Check sheet for the modelled part. Datum: model origin and axes. Units: mm. Coordinates: 2 decimals unless noted, no trailing zeros. Loops run counter-clockwise (first coordinate to the right, second up) from the corner with the lowest first, then second, coordinate; pieces in that order, holes last. Notation, with made-up numbers: (63, 21.5) -> (119, 21.5) arc R33 ccw to (119, 55.5) -> close; hole circle Ø8 at (-12.75, 6.5). An arc over 180 degrees is marked (long way). Use one line per item in the form item = value.
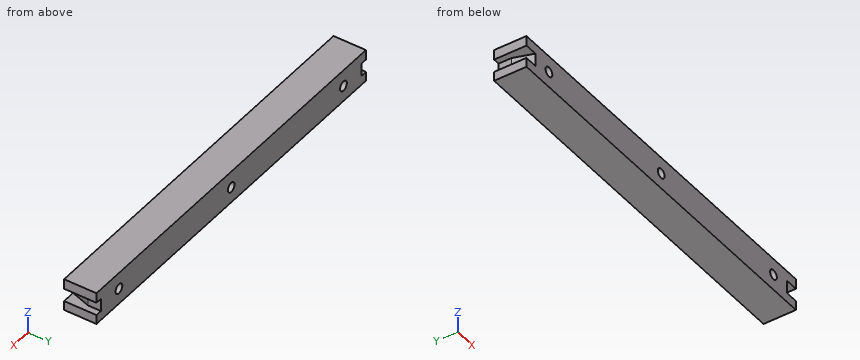
from build123d import *

# Parameters (mm, degrees)
ESQUISSE1_W                  = 120
ESQUISSE1_H                  = 10
ESQUISSE1_R                  = 1.5
BOSS_EXTRU_1_DEPTH           = 10
ENL_V_MAT_EXTRU_1_DEPTH      = 2
ENL_V_MAT_EXTRU_1_DEPTH_BACK = 2


with BuildPart() as part:
    # Esquisse1 → Boss.-Extru.1 (new body)
    with BuildSketch(Plane(origin=(0, 0, 0), x_dir=(1, 0, 0), z_dir=(0, 1, 0))):
        with Locations((0, -0.107913669)):
            Rectangle(ESQUISSE1_W, ESQUISSE1_H)
        with Locations((-50, 0)):
            Circle(ESQUISSE1_R, mode=Mode.SUBTRACT)
        Circle(ESQUISSE1_R, mode=Mode.SUBTRACT)
        with Locations((50, 0)):
            Circle(ESQUISSE1_R, mode=Mode.SUBTRACT)
    extrude(amount=BOSS_EXTRU_1_DEPTH)

    # Esquisse2 → Enlèv. mat.-Extru.1 (cut, two sides)
    with BuildSketch(Plane.XY) as enl_v_mat_extru_1_sk:
        Polygon((-58, 10), (-58, 6), (-56, 0), (-56, -10.800752999), (-73.153181154, -10.800752999), (-73.153181154, 18.339979991), (-58, 18.339979991), align=None)
        Polygon((58, 10), (58, 6), (56, 0), (56, -10.800752999), (73.153181154, -10.800752999), (73.153181154, 18.339979991), (58, 18.339979991), align=None)
    extrude(amount=ENL_V_MAT_EXTRU_1_DEPTH, mode=Mode.SUBTRACT)
    extrude(enl_v_mat_extru_1_sk.sketch, amount=-ENL_V_MAT_EXTRU_1_DEPTH_BACK, mode=Mode.SUBTRACT)


solid = part.part
(1) Section check B-B, the plane z = 0. Record the boundary of the cut face in (x, y), plus the area to 3 significant figures.
Established:
outline = (-58, 6) -> (-56, 0) -> (-51.5, 0) -> (-51.5, 10) -> (-58, 10) -> close; (-48.5, 0) -> (-1.5, 0) -> (-1.5, 10) -> (-48.5, 10) -> close; (1.5, 0) -> (48.5, 0) -> (48.5, 10) -> (1.5, 10) -> close; (51.5, 0) -> (56, 0) -> (58, 6) -> (58, 10) -> (51.5, 10) -> close
area = 1,060 mm²
(2) Go/stop test with a flat-tipped pin: P1, Ø2.5, axis at x = 0, z = 0, coming from the -Y side. Record where the tip stops, or that it passes through.
Established:
P1 = through
(3) Section check C-C, the plane y = 7. Record the boundary of the cut face in (x, z), plus the area to 3 significant figures.
Established:
outline = (-60, -4.89) -> (60, -4.89) -> (60, -2) -> (58, -2) -> (58, 2) -> (60, 2) -> (60, 5.11) -> (-60, 5.11) -> (-60, 2) -> (-58, 2) -> (-58, -2) -> (-60, -2) -> close; hole circle Ø3 at (-50, 0); hole circle Ø3 at (0, 0); hole circle Ø3 at (50, 0)
area = 1,160 mm²
(4) Scan lines: line 1 along X through (y, z) = (6.5, 0); line 2 along X through (y, z) = (4.5, 0.5); line 3 along Z through (x, y) = (-50, 4). Record each from-to range of solid material in increasing order.
Established:
line_1 = -58 to -51.5, -48.5 to -1.5, 1.5 to 48.5, 51.5 to 58
line_2 = -57.5 to -51.41, -48.59 to -1.41, 1.41 to 48.59, 51.41 to 57.5
line_3 = -4.89 to -1.5, 1.5 to 5.11
(5) Section check A-A, the plane x = 50. Record the boundary of the cut face in (y, z), plus the area to 3 significant figures.
Established:
outline = (0, -4.89) -> (10, -4.89) -> (10, -1.5) -> (0, -1.5) -> close; (0, 1.5) -> (10, 1.5) -> (10, 5.11) -> (0, 5.11) -> close
area = 70.0 mm²
(6) Section check D-D, the plane y = 2. Record the boundary of the cut face in (x, z), plus the area to 3 significant figures.
Established:
outline = (-60, -4.89) -> (60, -4.89) -> (60, -2) -> (56.67, -2) -> (56.67, 2) -> (60, 2) -> (60, 5.11) -> (-60, 5.11) -> (-60, 2) -> (-56.67, 2) -> (-56.67, -2) -> (-60, -2) -> close; hole circle Ø3 at (-50, 0); hole circle Ø3 at (0, 0); hole circle Ø3 at (50, 0)
area = 1,150 mm²
